Geometry check sheet. Reference: the model listing, model coordinates, mm. Face numbers are marked on the shaded views. A direction names the side the tool comes from. Give positions to 0.01 mm unless a question says otherwise; leave off trailing zeros. Order: outer loops, then holes, each group sorted by start corner. A loop starts at its lowest first (then second) coordinate and runs counter-clockwise, first axis right, second up. Notation, with made-up numbers: M 27,23 L 65,23 A34 cw 65,59 Z; hole C 41,61.25 d4. An arc over 180 degrees is marked long. Use CSV: the item, a comma, the result in double quotes. Start each with the question number.
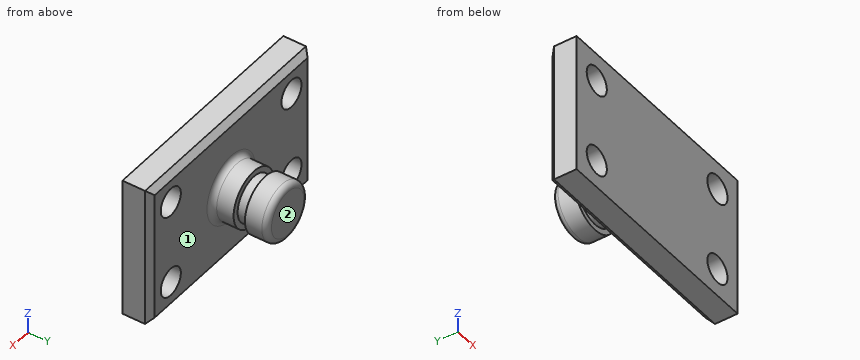
from build123d import *

# Parameters (mm, degrees)
F0_W     = 101.6
F0_H     = 63.5
F1_DEPTH = 12.7
F2_R     = 6.35
F3_DEPTH = 12.701
F4_W     = 12.7
F4_H     = 25.4
F6_W     = 9.067975
F6_H     = 5.08
F8_R     = 2.54
F9_SIZE  = 2.54


with BuildPart() as f1:
    # F0 (on Front) → F1 (new body)
    with BuildSketch(Plane.XZ):
        Rectangle(F0_W, F0_H)
    extrude(amount=-F1_DEPTH)

    # F2 (on face) → F3 (cut, through all)
    with BuildSketch(Plane(origin=(0, 12.7, 0), x_dir=(-1, 0, 0), z_dir=(0, 1, 0))):
        with Locations((38.1, -19.05)):
            Circle(F2_R)
        with Locations((-38.1, -19.05)):
            Circle(F2_R)
        with Locations((38.1, 19.05)):
            Circle(F2_R)
        with Locations((-38.1, 19.05)):
            Circle(F2_R)
    extrude(amount=-F3_DEPTH, mode=Mode.SUBTRACT)

    # F4 (on Top) → F5 (revolve)
    with BuildSketch(Plane.XY):
        with Locations((6.35, 25.4)):
            Rectangle(F4_W, F4_H)
    revolve(axis=Axis((0, 25.4, 0), (0, 1, 0)))

    # F6 (on Top) → F7 (revolve, cut)
    with BuildSketch(Plane.XY):
        with Locations((-14.693988, 25.4)):
            Rectangle(F6_W, F6_H)
    revolve(axis=Axis((0, 12.7, 0), (0, 1, 0)), mode=Mode.SUBTRACT)

    # F8
    f8_edges = [f1.edges().sort_by_distance(p)[0] for p in [
        (-12.7, 12.7, 0),
        (-12.7, 38.1, 0),
    ]]
    fillet(f8_edges, radius=F8_R)

    # F9
    f9_edges = [f1.edges().sort_by_distance(p)[0] for p in [
        (0, 12.7, -31.75),
        (50.8, 12.7, 0),
        (0, 12.7, 31.75),
        (-50.8, 12.7, 0),
    ]]
    chamfer(f9_edges, length=F9_SIZE)


solid = f1.part
(1) Sectioned sample at C-C on z = -19.05. Record the cut outline in (x, y), then the cut area to 3 significant figures.
(2) Access from +Z, -Z, +X, -X, +Y, -Y to the whole of each face (thin tool, end or side, straight path). Record for the marked faces 1 and 2.
(3) Sectioned sample at A-A on y = 11.5. Record the cut outline in (x, z), then the cut area to 3 significant figures.
(4) Thickness scan on line 1 (X direction, y = 3, z = -19); line 2 (Z direction, x = 38.1, y = 6); line 3 (Z direction, x = 33.5, y = 11.5). Record the ranges inside material, lowest first.
(5) Go/stop test with flat-tipped pins: P1, Ø8, axis at y = 23.5, z = -18.5, coming from the -X side; P2, Ø4, axis at x = -0.5, z = 18, coming from the +Y side; P3, Ø1.5, axis at y = 15, z = -7.5, coming from the -X side; P4, Ø4, axis at y = 14, z = 4.5, coming from the -X side. Record where each tip stops, or that it passes through.
(6) Sectioned sample at B-B on x = 38.1. Record the cut outline in (y, z).
(7) Sectioned sample at D-D on z = 0. Record the cut outline in (x, y).
Responses:
1,outline,"M -50.8,0 L -44.45,0 L -44.45,12.7 L -48.26,12.7 L -50.8,10.16 Z; M -31.75,0 L 31.75,0 L 31.75,12.7 L -31.75,12.7 Z; M 44.45,0 L 50.8,0 L 50.8,10.16 L 48.26,12.7 L 44.45,12.7 Z"
1,area,"961 mm2"
2,face 1,"+Y"
2,face 2,"+Z, -Z, +X, -X, +Y"
3,outline,"M -49.46,-30.41 L 49.46,-30.41 L 49.46,30.41 L -49.46,30.41 Z; hole C -38.1,-19.05 d12.7; hole C -38.1,19.05 d12.7; hole C 38.1,-19.05 d12.7; hole C 38.1,19.05 d12.7"
3,area,"5,510 mm2"
4,line 1,"-50.8 to -44.45, -31.75 to 31.75, 44.45 to 50.8"
4,line 2,"-31.75 to -25.4, -12.7 to 12.7, 25.4 to 31.75"
4,line 3,"-30.41 to -23.43, -14.67 to 14.67, 23.43 to 30.41"
5,P1,"through"
5,P2,"y = 12.7"
5,P3,"x = -10.79"
5,P4,"x = -48.96"
6,outline,"M 0,-31.75 L 10.16,-31.75 L 12.7,-29.21 L 12.7,-25.4 L 0,-25.4 Z; M 0,-12.7 L 12.7,-12.7 L 12.7,12.7 L 0,12.7 Z; M 0,25.4 L 12.7,25.4 L 12.7,29.21 L 10.16,31.75 L 0,31.75 Z"
7,outline,"M -50.8,0 L 50.8,0 L 50.8,10.16 L 48.26,12.7 L 15.24,12.7 A2.54 cw 12.7,15.24 L 12.7,22.86 L 10.16,22.86 L 10.16,27.94 L 12.7,27.94 L 12.7,35.56 A2.54 ccw 10.16,38.1 L -10.16,38.1 A2.54 ccw -12.7,35.56 L -12.7,27.94 L -10.16,27.94 L -10.16,22.86 L -12.7,22.86 L -12.7,15.24 A2.54 cw -15.24,12.7 L -48.26,12.7 L -50.8,10.16 Z"
